from build123d import *

# Parameters (mm, degrees)
F0_R     = 24
F0_R_2   = 11
F1_DEPTH = 12
F2_R     = 24
F2_R_2   = 11
F3_DEPTH = 16
F4_R     = 24
F4_R_2   = 11
F5_DEPTH = 12


with BuildPart() as f1:
    # F0 (on Front) → F1 (new body)
    with BuildSketch(Plane.XZ):
        Circle(F0_R)
        Circle(F0_R_2, mode=Mode.SUBTRACT)
    extrude(amount=F1_DEPTH)

    # F2 (on face) → F3 (join)
    with BuildSketch(Plane.XZ.offset(12)):
        Circle(F2_R)
        Circle(F2_R_2, mode=Mode.SUBTRACT)
    extrude(amount=F3_DEPTH)

    # F4 (on face) → F5 (join)
    with BuildSketch(Plane.XZ.offset(28)):
        Circle(F4_R)
        Circle(F4_R_2, mode=Mode.SUBTRACT)
    extrude(amount=F5_DEPTH)


solid = f1.part
For this review, take the finished solid that the model builds, in its own axes (mm). Give positions to 0.01 mm unless a question says otherwise; leave off trailing zeros. Order: outer loops, then holes, each group sorted by start corner. A loop starts at its lowest first (then second) coordinate and runs counter-clockwise, first axis right, second up. Notation, with made-up numbers: M 72,-8.75 L 101,-8.75 A20 ccw 101,-3.75 Z; hole C 44.5,58.25 d6. An arc over 180 degrees is marked long. Answer in a Markdown table with one row per item. Add a question column.
(1) Consider section B-B on z = 0. State the section outline as (x, y) points, and give its area (3 significant figures).
(2) Mouldability with a two-part tool opening along X and no side actions: class faces 1 (the face through (-23.977, -19.72, 1.055)), 2 (the face through (-2.38, -19.72, -10.74)), 3 (the face through (10, 0, -5)) as +X half, -X half, draft (parallel to the pull), parting line (faces both ways), or undercut.
(3) For pin 1 (12 mm diameter, centred on y = -6.5, z = -10, fed in from +X); pin 2 (10 mm diameter, centred on y = -9.5, z = -10.5, fed in from +X); pin 3 (6 mm diameter, centred on x = 9, y = -33.5, fed in from -Z), all flat-tipped, find the tip position at first contact; note any pin that passes through.
(4) Consider section D-D on x = 21.5. State the section outline as (y, z) points, and give its area (3 significant figures).
(5) Consider section A-A on x = 0. State the section outline as (y, z) points, and give its area (3 significant figures).
(6) Consider section C-C on y = -17. State the section outline as (x, z) points, and give its area (3 significant figures).
(7) Wall thickness on probe 1 along Z at (x, y) = (0, -27.5); probe 2 along X at (y, z) = (-16, 4.5); probe 3 along Z at (x, y) = (7, -12.5): over which ranges is each line inside the solid? List them lowest first. Write a range as [from, to].
Evaluation:
| question | item | result |
|---|---|---|
| 1 | outline | M -24,-40 L -11,-40 L -11,0 L -24,0 Z; M 11,-40 L 24,-40 L 24,0 L 11,0 Z |
| 1 | area | 1,040 mm^2 |
| 2 | face 1 | parting line |
| 2 | face 2 | undercut |
| 2 | face 3 | draft |
| 3 | pin 1 | stops at x = 23.66 |
| 3 | pin 2 | stops at x = 23.36 |
| 3 | pin 3 | stops at z = -23.24 |
| 4 | outline | M -40,-10.67 L 0,-10.67 L 0,10.67 L -40,10.67 Z |
| 4 | area | 853 mm^2 |
| 5 | outline | M -40,-24 L 0,-24 L 0,-11 L -40,-11 Z; M -40,11 L 0,11 L 0,24 L -40,24 Z |
| 5 | area | 1,040 mm^2 |
| 6 | outline | C 0,0 d48; hole C 0,0 d22 |
| 6 | area | 1,430 mm^2 |
| 7 | probe 1 | z = [-24, -11], [11, 24] |
| 7 | probe 2 | x = [-23.57, -10.04], [10.04, 23.57] |
| 7 | probe 3 | z = [-22.96, -8.49], [8.49, 22.96] |
